Model file for the job. Use its own axes, mm. A direction names the side the tool comes from. Coordinates: 2 decimals unless noted, no trailing zeros. Order: outer loops, then holes, each group sorted by start corner. A loop starts at its lowest first (then second) coordinate and runs counter-clockwise, first axis right, second up. Notation, with made-up numbers: (21, -32.75) -> (52, -32.75) arc R27 ccw to (52, -5.75) -> close; hole circle Ø7 at (35.5, -23.75). An arc over 180 degrees is marked (long way). Write item = value, one per line. Start each with the question number.
Q1. Mould opens along Z. For faces 5 (the face through (29, 29, -30.37)), 6 (the face through (13.58, 28.6, 0.18)), 7 (the face through (30, 23, 25)), 8 (the face through (15.54, 25.42, 16.95)) say: +Z half, -Z half, draft (parallel to the pull), parting line (faces both ways), or undercut.
Q2. Cut at B-B, the plane y = 25.31. List the corners of the cut face in (x, z).
Q3. Cut at A-A, the plane z = -25.37. List the corners of the cut face in (x, y), plus the area to 3 significant figures.
Q4. Wall check: line 1 (Z direction, x = 30.95, y = 25.31); line 2 (Z direction, x = 26.25, y = 17); line 3 (Y direction, x = 30.75, z = 25.37). Give the ranges that are in metal, low to high. Write a range as from..to.
Q5. Cut at C-C, the plane x = 27. List the corners of the cut face in (y, z), plus the area to 3 significant figures.
Q6. Flat gauge pins, fed straight in: pin 1 (2.5 mm diameter, centred on x = 27, z = -27, fed in from -Y); pin 2 (1 mm diameter, centred on y = 29, z = -27.5, fed in from -X); pin 3 (2.5 mm diameter, centred on y = 23, z = -25.5, fed in from -X). Where does each tip first touch, or does it go through?
Q7. 3-axis set-ups, long thin cutter, end or side, ignore diameter. For faces 1 (the face through (31, 20.31, -25)), 2 (the face through (22, 29, 25)), 3 (the face through (27, 20, 18.37)), 4 (the face through (25, 28.31, 25)): which of +Z, -Z, +X, -X, +Y, -Y reach the whole face in a straight line?
Autodesk Inventor part; units mm, degrees
ref_plane "YZ Plane" through (0, 0, 0) normal (1, 0, 0) x (0, 1, 0)
ref_plane "XZ Plane" through (0, 0, 0) normal (0, 1, 0) x (-1, 0, 0)
ref_plane "XY Plane" through (0, 0, 0) normal (0, 0, 1) x (1, 0, 0)
sketch "Boceto1" plane through (0, 0, 0) normal (0, 1, 0) x (-1, 0, 0)
  line L0 (-18.96, -20.37) -> (-32, -20.37)
  line L1 (-32, -20.37) -> (-32, 20.37)
  line L2 (-32, 20.37) -> (-18.96, 20.37)
  line L3 (-18.96, 20.37) -> (-10, 11.41)
  line L4 (-18.96, -20.37) -> (-10, -11.41)
  line L5 (-10, 0) -> (-10, 14.0554)
  line L6 (-10, 0) -> (4.0554, 0) construction
  line L7 (-10, 14.0554) -> (-10, -14.0554)
  dimension "d15" = 13.04
  dimension "d16" = 40.74
  dimension "d17" = 13.04
  dimension "d108" = 90
extrude "Extrusión1" add sketch "Boceto1" along normal blind 20.31
sketch "Boceto7" plane through (0, 20.31, 0) normal (0, 1, 0) x (1, 0, 0)
  line L0 (6.8202, -5.4018) -> (6.8202, 5.4018)
  line L1 (32, -20.37) -> (32, 20.37)
  line L2 (32, 20.37) -> (18.96, 20.37)
  line L3 (18.96, 20.37) -> (10, 11.41)
  line L4 (10, -11.41) -> (18.96, -20.37)
  line L5 (18.96, -20.37) -> (32, -20.37)
  line L6 (10, 11.41) -> (10, -11.41)
  point P0 (0, 0)
extrude "Extrusión5" add sketch "Boceto7" along normal blind 10
chamfer "Chaflán2" distance 30.31 distance2 22 1 edges at (10, 0, 0) measured on face at (10, 10.1033, -3.8033)
shell "Vaciado2" thickness 2 removed faces 3 at (24.6667, 30.31, 3.8033) at (32, 0, 6.79) at (32, 10.1033, 6.79)
chamfer "Chaflán3" distance 2 angle 45 1 edges at (12.4712, 30.31, 0)
fillet "Empalme2" radius 4 1 edges at (13.646, 28.6914, 0)
sketch "Boceto13" plane through (18.96, 30.31, 20.37) normal (0, 0, 1) x (1, 0, 0)
  line L0 (13.04, 0) -> (3.04, 0)
  line L1 (3.04, 0) -> (3.04, -2)
  line L2 (3.04, -2) -> (13.04, -2)
  line L3 (13.04, -2) -> (13.04, 0)
  line L4 (13.04, 0) -> (11.04, 0)
  line L5 (11.04, 0) -> (11.04, -10)
  line L6 (11.04, -10) -> (13.04, -10)
  line L7 (13.04, -10) -> (13.04, 0)
  point P0 (-18.96, -30.31)
  point P1 (11.04, -2)
  point P2 (13.04, -2)
  dimension "d123" = 10
  dimension "d124" = 2
  dimension "d125" = 2
  dimension "d126" = 10
extrude "Extrusión9" add sketch "Boceto13" along normal blind 10
sketch "Boceto14" plane through (32, 30.31, -20.37) normal (0, 0, -1) x (-1, 0, 0)
  line L0 (0, -26.9052) -> (0, 0)
  line L1 (0, 0) -> (10, 0)
  line L2 (10, 0) -> (10, -2)
  line L3 (10, -2) -> (0, -2)
  line L4 (0, -2) -> (0, 0)
  line L5 (0, 0) -> (12.2116, 0)
  line L6 (0, 0) -> (2, 0)
  line L7 (2, 0) -> (2, -10)
  line L8 (2, -10) -> (0, -10)
  line L9 (0, -10) -> (0, 0)
  point P0 (32, -30.31)
  point P1 (2, -2)
  dimension "d129" = 10
  dimension "d130" = 2
  dimension "d131" = 2
  dimension "d132" = 10
extrude "Extrusión10" add sketch "Boceto14" along normal blind 10
sketch "Boceto15" plane through (32, 0, 20.37) normal (1, 0, 0) x (0, 0, -1)
  line L0 (2, 30.31) -> (-10, 30.31)
  line L1 (-10, 20.31) -> (-10, 30.31)
  line L2 (38.74, 30.31) -> (50.74, 30.31)
  line L3 (50.74, 30.31) -> (50.74, 20.31)
  point P0 (20.37, 0)
  point P1 (-5, 25.31)
  point P2 (45.74, 25.31)
  dimension "d135" = 5
  dimension "d136" = 5
  dimension "d144" = 5
  dimension "d145" = 5
hole "Agujero5" at (32, 25.31, 25.37) at (32, 25.31, -25.37) direction (-1, 0, 0) diameter 2 depth 2.5 tip angle 118
sketch "Boceto16" plane through (0, 30.31, 0) normal (0, 1, 0) x (1, 0, 0)
  line L0 (32, -30.37) -> (22, -30.37)
  line L1 (22, -20.37) -> (22, -30.37)
  line L2 (22, 30.37) -> (32, 30.37)
  line L3 (22, 20.37) -> (22, 30.37)
  point P0 (0, 0)
  point P1 (27, -25.37)
  point P2 (27, 25.37)
  dimension "d146" = 5
  dimension "d147" = 5
  dimension "d148" = 5
  dimension "d149" = 5
hole "Agujero6" at (27, 30.31, 25.37) at (27, 30.31, -25.37) direction (0, -1, 0) diameter 2 depth 2.5 tip angle 118
properties part number "Rampa2"
Here are the results:
q1.face_5 = -Z half
q1.face_6 = undercut
q1.face_7 = draft
q1.face_8 = +Z half
q2.outline = (13.63, -15.04) -> (18.96, -20.37) -> (30, -20.37) -> (30, -24.37) -> (32, -24.37) -> (32, -18.37) -> (19.79, -18.37) -> (16.1, -14.68) -> (16.1, 14.68) -> (19.79, 18.37) -> (32, 18.37) -> (32, 24.37) -> (30, 24.37) -> (30, 20.37) -> (18.96, 20.37) -> (13.63, 15.04) -> close; (30, -30.37) -> (32, -30.37) -> (32, -26.37) -> (30, -26.37) -> close; (30, 26.37) -> (32, 26.37) -> (32, 30.37) -> (30, 30.37) -> close
q3.outline = (22, 28.31) -> (26, 28.31) -> (26, 30.31) -> (22, 30.31) -> close; (28, 28.31) -> (30, 28.31) -> (30, 26.31) -> (32, 26.31) -> (32, 30.31) -> (28, 30.31) -> close; (30, 20.31) -> (32, 20.31) -> (32, 24.31) -> (30, 24.31) -> close
q3.area = 28.0 mm²
q4.line_1 = -30.37..-26.37, -24.37..-18.37, 18.37..24.37, 26.37..30.37
q4.line_2 = -20.37..-18.37, 18.37..20.37
q4.line_3 = 20.31..24.31, 26.31..30.31
q5.outline = (6.89, -20.37) -> (28.31, -20.37) -> (28.31, -24.37) -> (30.31, -24.37) -> (30.31, -18.37) -> (10.29, -18.37) -> (10.29, 18.37) -> (30.31, 18.37) -> (30.31, 24.37) -> (28.31, 24.37) -> (28.31, 20.37) -> (6.89, 20.37) -> close; (28.31, -30.37) -> (30.31, -30.37) -> (30.31, -26.37) -> (28.31, -26.37) -> close; (28.31, 26.37) -> (30.31, 26.37) -> (30.31, 30.37) -> (28.31, 30.37) -> close
q5.area = 251 mm²
q6.pin_1 = 28.31
q6.pin_2 = 22
q6.pin_3 = 30
q7.face_1 = -Z, +X, -X, -Y
q7.face_2 = +Z, -X, +Y, -Y
q7.face_3 = +X, +Y
q7.face_4 = +Z, -X, -Y
